from build123d import *

# Parameters (mm, degrees)
F0_W     = 15.875
F0_H     = 15.875
F0_R     = 2.2550277878
F0_R_2   = 3.175
F0_R_3   = 2.38125
F1_DEPTH = 9.525
F2_DEPTH = 11.1125
F3_DEPTH = 9.525
F5_DEPTH = 25.4
F6_T     = -1.5875


with BuildPart() as f1:
    # F0 (on Top) → F1 (new body)
    with BuildSketch(Plane.XY):
        Rectangle(F0_W, F0_H)
        with Locations((-3.96875, 3.96875)):
            Circle(F0_R, mode=Mode.SUBTRACT)
        Circle(F0_R_2, mode=Mode.SUBTRACT)
        with Locations((3.96875, 3.96875)):
            Circle(F0_R, mode=Mode.SUBTRACT)
        Circle(F0_R_2)
        Circle(F0_R_3, mode=Mode.SUBTRACT)
        Circle(F0_R_3)
    extrude(amount=F1_DEPTH)

    # F0 (on Top) → F2 (join)
    with BuildSketch(Plane.XY):
        with Locations((-3.96875, 3.96875)):
            Circle(F0_R)
        with Locations((3.96875, 3.96875)):
            Circle(F0_R)
    extrude(amount=F2_DEPTH)

    # F0 (on Top) → F3 (join)
    with BuildSketch(Plane.XY):
        Circle(F0_R_2)
        Circle(F0_R_3, mode=Mode.SUBTRACT)
    extrude(amount=F3_DEPTH)

    # F4 (on face) → F5 (cut)
    with BuildSketch(Plane.YZ.offset(7.9375)):
        Polygon((-7.9375, 9.525), (-7.9375, 3.175), (0, 9.525), align=None)
    extrude(amount=-F5_DEPTH, mode=Mode.SUBTRACT)

    # F6
    f6_openings = [f1.faces().sort_by_distance(p)[0] for p in [
        (0, 0, 0),
    ]]
    offset(amount=F6_T, openings=f6_openings, kind=Kind.INTERSECTION)


solid = f1.part
Could you check a few things on this model? Use its own coordinates, in mm. A direction names the side the tool comes from. Give positions to 0.01 mm unless a question says otherwise; leave off trailing zeros. Order: outer loops, then holes, each group sorted by start corner. A loop starts at its lowest first (then second) coordinate and runs counter-clockwise, first axis right, second up.
1. Suppose I cut it at B-B (z = 5.25). List the corners of the cut face in (x, y) for me.
2. Suppose I cut it at D-D (z = 8.25). List the corners of the cut face in (x, y) for me, plus the area to 3 significant figures.
3. I need wall thicknesses on L1, parallel to X at y = -0.25, z = 6.5. Which ranges of the line are inside material? Lowest first, please.
4. For faces 4 (the flat face through (0.11, -4.02, 6.31)), 5 (the cylindrical face through (5.01, 1.97, 10.31)), 6 (the flat face through (0, 3, 7.938)), which set-ups out of +Z, -Z, +X, -X, +Y, -Y let a thin tool reach every point of the face, with its end or its side?
5. We'd pull the mould along Y, two halves only. Please class faces 1 (the flat face through (0.09, -2.94, 5.14)), 2 (the flat face through (0, -7.938, 2)), 3 (the flat face through (0, 4, 9.525)): pulls with the +Y half, pulls with the -Y half, needs draft (parallel to the pull), parting line crosses it, or undercut.
6. Will these pins go through, and if not, where does the flat tip stop? P1, Ø1, axis at x = 2, z = 4.5, coming from the -Y side; P2, Ø1.5, axis at x = -2, y = 1, coming from the +Z side (3 decimals); P3, Ø1, axis at x = 0, z = 8.5, coming from the -Y side.
Solved:
1. outline: (-7.94, -5.34) - (7.94, -5.34) - (7.94, 7.94) - (-7.94, 7.94) - close; hole (-6.35, -2.8) - (6.35, -2.8) - (6.35, 6.35) - (-6.35, 6.35) - close
2. outline: (-7.94, -1.59) - (7.94, -1.59) - (7.94, 7.94) - (-7.94, 7.94) - close; hole circle Ø1.34 at (-3.97, 3.97); hole circle Ø1.34 at (3.97, 3.97)
2. area: 149 mm2
3. L1: x = -7.94 to -6.35, 6.35 to 7.94
4. face 4: +Z, +X, -X, -Y
4. face 5: +Z
4. face 6: -Z
5. face 1: undercut
5. face 2: pulls with the -Y half
5. face 3: needs draft
6. P1: stops at y = -6.91
6. P2: stops at z = 9.525
6. P3: stops at y = -1.91
